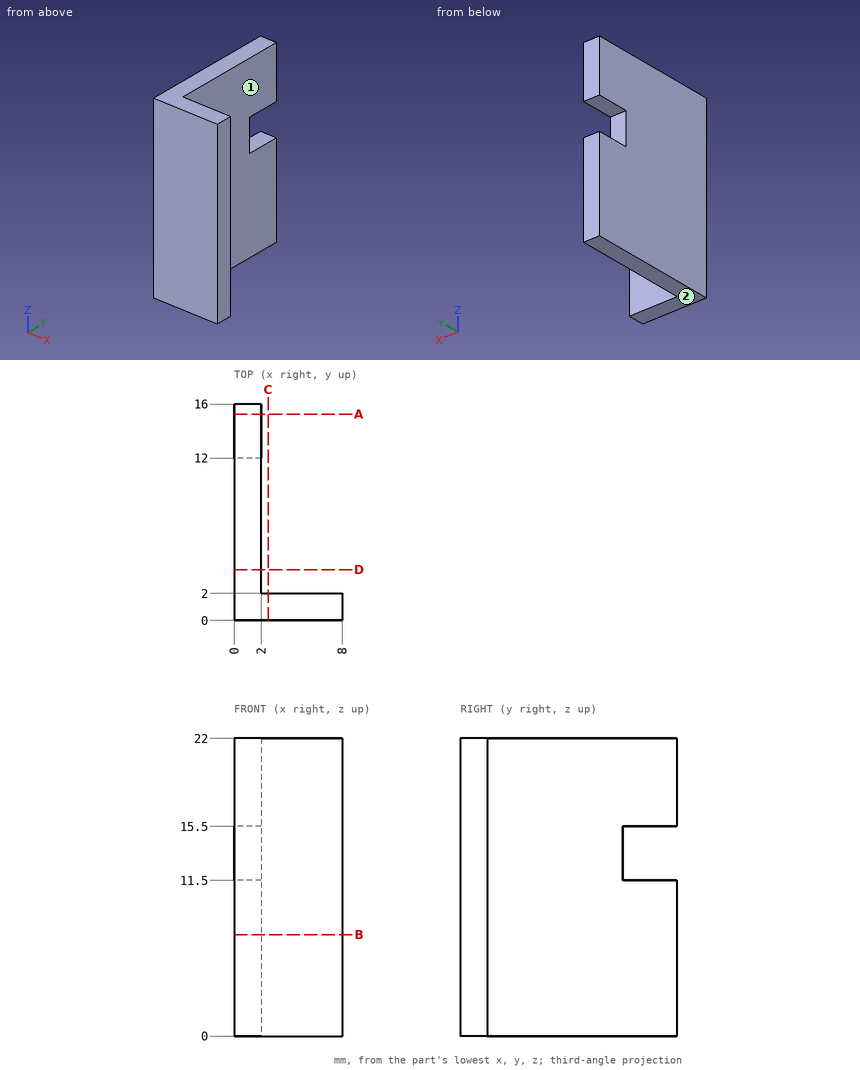
Answer from the drawing. Dimensions are ordinates in mm from the lowest x, y and z of the part. A direction names the side the tool comes from. Coordinates: 2 decimals unless noted, no trailing zeros. Order: outer loops, then holes, each group sorted by start corner. A loop starts at its lowest first (then second) coordinate and runs counter-clockwise, first axis right, second up. Notation, with made-up numbers: (74.25, -6) - (126.25, -6) arc R11 cw to (126.25, 9) - close; hole circle Ø1 at (-17.75, 87). An arc over 180 degrees is marked (long way). Put each result on its own line as item: value. Start each with the question number.
1) Find the intervals of material crossed by line 1 (X direction, y = 6.5, z = 11.25); line 2 (Y direction, x = 1, z = 13.5), in increasing order. Write a range as from..to.
2) Find section B-B (z = 7.5). Give the vertices of the cut face in (x, y), plus the area to 3 significant figures.
3) Flat-ended cylindrical pins translate along their axes: pin 1 (1 mm diameter, centred on y = 12.5, z = 8, fed in from +X); pin 2 (0.6 mm diameter, centred on x = 1, z = 13, fed in from +Y). Find the tip coordinate at first contact, or state that the pin passes through.
4) Find section C-C (x = 2.5). Give the vertices of the cut face in (y, z).
5) Find section A-A (y = 15.25). Give the vertices of the cut face in (x, z), plus the area to 3 significant figures.
6) For the marked faces 1 and 2, determine the directions among +Z, -Z, +X, -X, +Y, -Y from which every point of the face is accessible in a straight line to the end or side of a thin tool.
Results list:
1. line 1: x = 0..2
1. line 2: y = 0..12
2. outline: (0, 0) - (8, 0) - (8, 2) - (2, 2) - (2, 16) - (0, 16) - close
2. area: 44.0 mm^2
3. pin 1: stops at x = 2
3. pin 2: stops at y = 12
4. outline: (0, 0) - (2, 0) - (2, 22) - (0, 22) - close
5. outline: (0, 0) - (2, 0) - (2, 11.5) - (0, 11.5) - close; (0, 15.5) - (2, 15.5) - (2, 22) - (0, 22) - close
5. area: 36.0 mm^2
6. face 1: +Z, -Z, +X, +Y
6. face 2: -Z, +X, -X, +Y, -Y
